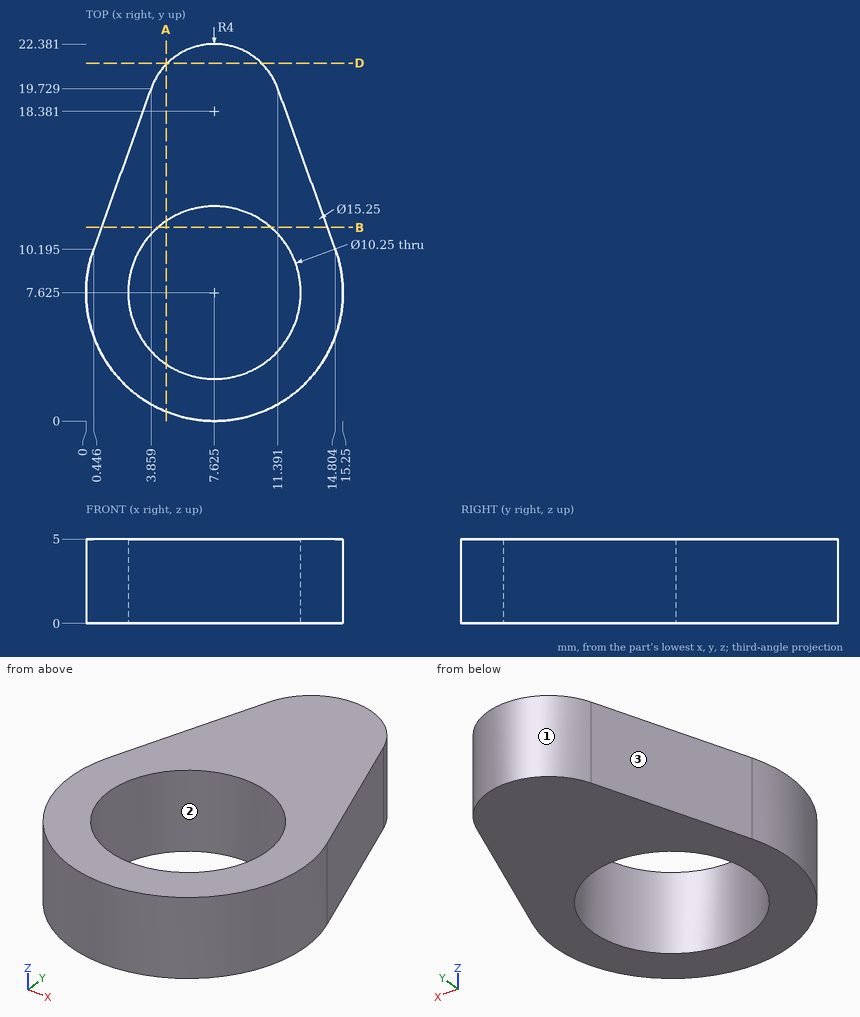
Can you work these out from the drawing? Everything is in mm from the part's minimum corner. Coordinates: 2 decimals unless noted, no trailing zeros. Loops run counter-clockwise (first coordinate to the right, second up) from the corner with the lowest first, then second, coordinate; pieces in that order, holes last. Notation, with made-up numbers: M 53,-1.5 L 63,-1.5 A11 ccw 63,19.5 Z; hole C 46.5,83.25 d7. An arc over 180 degrees is marked long. Put each result on its own line as item: value. Start each with the question number.
(1) I need wall thicknesses on line 1 (X direction, y = 8.25, z = 1.45) (1 decimal); line 2 (X direction, y = 5.5, z = 4); line 3 (Y direction, x = 6.5, z = 3.55) (1 decimal). Which ranges of each line are inside material? Lowest first, please. Write a range as from..to.
(2) Suppose I cut it at B-B on y = 11.5. Please give me the cut outline in (x, z).
(3) Thinking about a two-plate mould opening in X: for the marked faces 1, 2 and 3, which applies, pulls with the +X half, pulls with the -X half, needs draft (parallel to the pull), parting line crosses it, or undercut?
(4) Will this pin go through, and if not, where does the flat tip stop? P1, Ø1.5, axis at y = 17, z = 2.5, coming from the +X side.
(5) Suppose I cut it at D-D on y = 21.25. Please give me the cut outline in (x, z).
(6) Suppose I cut it at A-A on x = 4.75. Please give me the cut outline in (y, z).
Solutions:
1. line 1: x = 0..2.5, 12.7..15.2
1. line 2: x = 0.3..2.96, 12.29..14.95
1. line 3: y = 0.1..2.6, 12.6..22.2
2. outline: M 0.91,0 L 4.27,0 L 4.27,5 L 0.91,5 Z; M 10.98,0 L 14.34,0 L 14.34,5 L 10.98,5 Z
3. face 1: parting line crosses it
3. face 2: undercut
3. face 3: pulls with the -X half
4. P1: stops at x = 12.64
5. outline: M 4.84,0 L 10.41,0 L 10.41,5 L 4.84,5 Z
6. outline: M 0.56,0 L 3.38,0 L 3.38,5 L 0.56,5 Z; M 11.87,0 L 21.16,0 L 21.16,5 L 11.87,5 Z
